```python
from build123d import *

# Parameters (mm, degrees)
F0_R     = 76.2
F0_R_2   = 12.7
F1_DEPTH = 6.35


with BuildPart() as f1:
    # F0 (on Top) → F1 (new body)
    with BuildSketch(Plane.XY):
        Circle(F0_R)
        with Locations((-8.821327, -50.028234)):
            Circle(F0_R_2, mode=Mode.SUBTRACT)
        with Locations((-38.915058, -32.653611)):
            Circle(F0_R_2, mode=Mode.SUBTRACT)
        with Locations((25.4, -43.994091)):
            Circle(F0_R_2, mode=Mode.SUBTRACT)
        with Locations((47.736385, -17.374623)):
            Circle(F0_R_2, mode=Mode.SUBTRACT)
        with Locations((-50.8, 0)):
            Circle(F0_R_2, mode=Mode.SUBTRACT)
        with Locations((-38.915058, 32.653611)):
            Circle(F0_R_2, mode=Mode.SUBTRACT)
        with Locations((-8.821327, 50.028234)):
            Circle(F0_R_2, mode=Mode.SUBTRACT)
        Circle(F0_R_2, mode=Mode.SUBTRACT)
        with Locations((47.736385, 17.374623)):
            Circle(F0_R_2, mode=Mode.SUBTRACT)
        with Locations((25.4, 43.994091)):
            Circle(F0_R_2, mode=Mode.SUBTRACT)
    extrude(amount=F1_DEPTH)


solid = f1.part
```
Build history of the part. All positions in model axes, mm. Give positions to 0.01 mm unless a question says otherwise; leave off trailing zeros. Loops run counter-clockwise (first coordinate to the right, second up) from the corner with the lowest first, then second, coordinate; pieces in that order, holes last.
Item 1: Slice it at C-C, the plane x = 24. List the corners of the cut face in (y, z).
Answers follow:
outline: (-72.32, 0) - (-56.62, 0) - (-56.62, 6.35) - (-72.32, 6.35) - close; (-31.37, 0) - (31.37, 0) - (31.37, 6.35) - (-31.37, 6.35) - close; (56.62, 0) - (72.32, 0) - (72.32, 6.35) - (56.62, 6.35) - close
Item 2: Slice it at B-B, the plane x = 0. List the corners of the cut face in (y, z), and give its area (3 significant figures).
Answers follow:
outline: (-76.2, 0) - (-59.16, 0) - (-59.16, 6.35) - (-76.2, 6.35) - close; (-40.89, 0) - (-12.7, 0) - (-12.7, 6.35) - (-40.89, 6.35) - close; (12.7, 0) - (40.89, 0) - (40.89, 6.35) - (12.7, 6.35) - close; (59.16, 0) - (76.2, 0) - (76.2, 6.35) - (59.16, 6.35) - close
area: 574 mm2
Item 3: Slice it at A-A, the plane y = 0. List the corners of the cut face in (x, z), and give its area (3 significant figures).
Answers follow:
outline: (-76.2, 0) - (-63.5, 0) - (-63.5, 6.35) - (-76.2, 6.35) - close; (-38.1, 0) - (-12.7, 0) - (-12.7, 6.35) - (-38.1, 6.35) - close; (12.7, 0) - (76.2, 0) - (76.2, 6.35) - (12.7, 6.35) - close
area: 645 mm2
Item 4: Pull direction Y, two halves, no side cores. Call faces 1 (the face through (-40.57, -20.06, 3.13)), 2 (the face through (-1, -16, 0)), 3 (the face through (-60.47, -46.367, 3.131)): released by +Y, released by -Y, zero draft, split by the parting line, or undercut.
Answers follow:
face 1: undercut
face 2: zero draft
face 3: split by the parting line
Item 5: Drill centre lines: line 1 (Y direction, x = -44, z = 4.25); line 2 (Y direction, x = 0, z = 2); line 3 (Y direction, x = 20, z = 5.75). Where is each one in solid material? Low to high.
Answers follow:
line 1: y = -62.21 to -44.29, -21.02 to -10.73, 10.73 to 21.02, 44.29 to 62.21
line 2: y = -76.2 to -59.16, -40.89 to -12.7, 12.7 to 40.89, 59.16 to 76.2
line 3: y = -73.53 to -55.49, -32.5 to 32.5, 55.49 to 73.53
Item 6: Flat gauge pins, fed straight in: pin 1 (1.5 mm diameter, centred on x = 24.5, z = 0.5, fed in from +Y); pin 2 (1.5 mm diameter, centred on x = 41.5, z = 1, fed in from -Y); pin 3 (1 mm diameter, centred on y = -23.5, z = 2, fed in from +X); pin 4 (23 mm diameter, centred on x = -38.92, y = 32.65, fed in from -Z). Where does each tip first touch, or does it go through?
Answers follow:
pin 1: stops at y = 72.4
pin 2: stops at y = -64.39
pin 3: stops at x = 72.65
pin 4: passes through
Item 7: Slice it at D-D, the plane z = 2.5. Give the number of separate pieces and of enclosed holes in the cut face, and give its area (3 significant figures).
Answers follow:
separate pieces: 1
enclosed holes: 10
area: 13,200 mm2
